Autodesk Fusion 360 part; units mm, degrees
sketch "Esquisse1" plane through (0, 0, 0) normal (0, 0, 1) x (1, 0, 0)
  line L0 (-37.7016, 28.5178) -> (39.7984, 28.5178)
  line L1 (39.7984, 28.5178) -> (39.7984, -27.4822)
  line L2 (39.7984, -27.4822) -> (-37.7016, -27.4822)
  line L3 (-37.7016, -27.4822) -> (-37.7016, 28.5178)
  dimension "d1" = 77.5
  dimension "d2" = 56
extrude "Extrusion1" add sketch "Esquisse1" along normal blind 19
sketch "Esquisse2" plane through (0, 0, 19) normal (0, 0, 1) x (-1, 0, 0)
  line L0 (37.7016, 27.4822) -> (-39.7984, 27.4822)
  line L1 (-39.7984, 27.4822) -> (-39.7984, -28.5178)
  line L2 (-39.7984, -28.5178) -> (37.7016, -28.5178)
  line L3 (37.7016, -28.5178) -> (37.7016, 27.4822)
  line L4 (-39.2984, -28.0178) -> (37.2016, -28.0178)
  line L5 (37.2016, -28.0178) -> (37.2016, 26.9822)
  line L6 (37.2016, 26.9822) -> (-39.2984, 26.9822)
  line L7 (-39.2984, 26.9822) -> (-39.2984, -28.0178)
  dimension "d5" = -0.5
extrude "Extrusion2" cut sketch "Esquisse2" against normal blind 15 contours L4 L5 L6 L7
sketch "Esquisse5" plane through (0, 0, 4) normal (0, 0, 1) x (-1, 0, 0)
  line L0 (-39.2984, 26.9822) -> (-39.2984, -28.0178)
  line L1 (-39.2984, -28.0178) -> (37.2016, -28.0178)
  line L2 (37.2016, -28.0178) -> (37.2016, 26.9822)
  line L3 (37.2016, 26.9822) -> (-39.2984, 26.9822)
  line L4 (37.7016, 27.4822) -> (-39.7984, 27.4822)
  line L5 (-39.2984, 26.9822) -> (37.2016, 26.9822)
  line L6 (37.2016, -28.0178) -> (-39.2984, -28.0178)
  line L7 (-39.7984, -28.5178) -> (37.7016, -28.5178)
  line L8 (-24.7984, 27.4822) -> (-11.7984, 27.4822)
  line L9 (-11.7984, 27.4822) -> (-11.7984, 26.9822)
  line L10 (-11.7984, 26.9822) -> (-24.7984, 26.9822)
  line L11 (-24.7984, 26.9822) -> (-24.7984, 27.4822)
  line L12 (9.7016, -28.0178) -> (22.7016, -28.0178)
  line L13 (22.7016, -28.0178) -> (22.7016, -28.5178)
  line L14 (22.7016, -28.5178) -> (9.7016, -28.5178)
  line L15 (9.7016, -28.5178) -> (9.7016, -28.0178)
  line L16 (-39.7984, 27.4822) -> (-39.7984, -28.5178)
  line L17 (-39.2984, -28.0178) -> (-39.2984, 26.9822)
  line L18 (37.2016, 26.9822) -> (37.2016, -28.0178)
  line L19 (37.7016, -28.5178) -> (37.7016, 27.4822)
  dimension "d11" = 13
  dimension "d12" = 13
  dimension "d13" = 15
  dimension "d14" = 15
extrude "Extrusion3" add sketch "Esquisse5" along normal blind 16.5 contours L3 L4 L5 L8 L9 L10 L11 | L1 L6 L7 L12 L13 L14 L15
sketch "Esquisse6" plane through (0, 0, 4) normal (0, 0, 1) x (-1, 0, 0)
  line L0 (-39.2984, 26.9822) -> (-39.2984, -28.0178)
  line L1 (-39.2984, -28.0178) -> (37.2016, -28.0178)
  line L2 (37.2016, -28.0178) -> (37.2016, 26.9822)
  line L3 (37.2016, 26.9822) -> (-39.2984, 26.9822)
  circle A0 centre (14.7016, -24.5178) radius 1
  circle A1 centre (17.2016, 23.4822) radius 1
  line L4 (37.7016, -28.5178) -> (37.7016, 27.4822)
  line L5 (9.7016, -28.5178) -> (22.7016, -28.5178)
  line L6 (37.7016, 27.4822) -> (-11.7984, 27.4822)
  dimension "d17" = 2
  dimension "d18" = 2
  dimension "d22" = 4
  dimension "d23" = 4
  dimension "d49" = 20
  dimension "d50" = 22.5
extrude "Extrusion4" add sketch "Esquisse6" along normal blind 6 contours A0 | A1
sketch "Esquisse7" plane through (-37.7016, 0, 0) normal (-1, 0, 0) x (0, -1, 0)
  line L0 (-28.5178, 0) -> (27.4822, 0)
  line L1 (27.4822, 0) -> (27.4822, 19)
  line L2 (27.4822, 19) -> (-28.5178, 19)
  line L3 (-28.5178, 19) -> (-28.5178, 0)
  line L4 (-18.5178, 10.6) -> (-6.5178, 10.6)
  line L5 (-6.5178, 10.6) -> (-6.5178, 3.1)
  line L6 (-6.5178, 3.1) -> (-18.5178, 3.1)
  line L7 (-18.5178, 3.1) -> (-18.5178, 10.6)
  line L8 (13.4822, 17.1) -> (21.9822, 17.1)
  line L9 (21.9822, 17.1) -> (21.9822, 4.1)
  line L10 (21.9822, 4.1) -> (13.4822, 4.1)
  line L11 (13.4822, 4.1) -> (13.4822, 17.1)
  dimension "d26" = 12
  dimension "d27" = 7.5
  dimension "d28" = 10
  dimension "d29" = 8.5
  dimension "d30" = 13
  dimension "d31" = 5.5
  dimension "d32" = 4.1
  dimension "d33" = 3.1
extrude "Extrusion5" cut sketch "Esquisse7" against normal blind 33 contours L4 L5 L6 L7 | L8 L9 L10 L11
extrude "Extrusion6" cut sketch "Esquisse6" against normal blind 3
extrude "Extrusion7" add 1 faces at (-11.8683, 9.8511, 0) along direction (0, 0, -1) blind 2
sketch "Esquisse8" plane through (0, 0, 0) normal (0, 0, 1) x (1, 0, 0)
  line L0 (39.7984, 28.5178) -> (-9.7016, 28.5178)
  line L1 (-9.7016, 28.5178) -> (-22.7016, 28.5178)
  line L2 (-22.7016, 28.5178) -> (-37.7016, 28.5178)
  line L3 (-37.7016, 28.5178) -> (-37.7016, -27.4822)
  line L4 (39.7984, -27.4822) -> (39.7984, 28.5178)
  line L5 (24.7984, -27.4822) -> (39.7984, -27.4822)
  line L6 (11.7984, -27.4822) -> (24.7984, -27.4822)
  line L7 (-37.7016, -27.4822) -> (11.7984, -27.4822)
  line L8 (24.7984, -29.4822) -> (41.7984, -29.4822)
  line L9 (41.7984, -29.4822) -> (41.7984, 30.5178)
  line L10 (41.7984, 30.5178) -> (-9.7016, 30.5178)
  line L11 (-9.7016, 30.5178) -> (-22.7016, 30.5178)
  line L12 (-22.7016, 30.5178) -> (-39.7016, 30.5178)
  line L13 (-39.7016, 30.5178) -> (-39.7016, -29.4822)
  line L14 (-39.7016, -29.4822) -> (11.7984, -29.4822)
  line L15 (11.7984, -29.4822) -> (24.7984, -29.4822)
  dimension "d40" = 2
extrude "Extrusion8" add sketch "Esquisse8" along normal blind 24 and the other way blind 2
extrude "Extrusion9" cut 2 faces at (-37.7016, -16.3155, 8.4333) (-37.7016, 14.5178, 5.6) along direction (1, 0, 0) blind 0 and the other way blind 5
extrude "Extrusion10" add sketch "Esquisse6" along normal blind 6 and the other way blind 2 contours A1
sketch "Esquisse9" plane through (39.7984, 0, 0) normal (-1, 0, 0) x (0, -1, 0)
  line L0 (-28.5178, 19) -> (27.4822, 19)
  line L1 (27.4822, 19) -> (27.4822, 24)
  line L2 (27.4822, 24) -> (-28.5178, 24)
  line L3 (-28.5178, 24) -> (-28.5178, 19)
  line L4 (12.4822, 24) -> (22.4822, 24)
  line L5 (22.4822, 24) -> (22.4822, 23.3)
  line L6 (22.4822, 23.3) -> (12.4822, 23.3)
  line L7 (12.4822, 23.3) -> (12.4822, 24)
  dimension "d55" = 10
  dimension "d56" = 0.7
  dimension "d57" = 5
extrude "Extrusion11" add sketch "Esquisse9" along normal blind 2 contours L2 L4 L5 L6 L7
sketch "Esquisse10" plane through (-37.7016, 0, 0) normal (1, 0, 0) x (0, 1, 0)
  line L0 (-27.4822, 19) -> (28.5178, 19)
  line L1 (28.5178, 19) -> (28.5178, 24)
  line L2 (28.5178, 24) -> (-27.4822, 24)
  line L3 (-27.4822, 24) -> (-27.4822, 19)
  line L4 (-27.4822, 24) -> (-17.4822, 24)
  line L5 (-17.4822, 24) -> (-17.4822, 23.3)
  line L6 (-17.4822, 23.3) -> (-27.4822, 23.3)
  line L7 (-27.4822, 23.3) -> (-27.4822, 24)
  dimension "d60" = 10
  dimension "d61" = 0.7
extrude "Extrusion12" add sketch "Esquisse10" along normal blind 2 contours L2 L3 L4 L5 L6 L7
fillet "Congé1" radius 0.45 4 edges at (41.7984, -29.4822, 11) (41.7984, 30.5178, 11) (-39.7016, 30.5178, 11) (-39.7016, -29.4822, 11)
equation "d1 = LongueurBoite"
equation "d2 = LargeurBoite"
equation "d26 = LargeurTrouUSB"
equation "d27 = HauteurTrouUSB"
equation "d28 = DistanceBordTrouUSB"
equation "d29 = LargeurTrouAC"
equation "d30 = HauteurTrouAC"
equation "d31 = DistanceBordTrouAC"
equation "d32 = DistanceDessousTrouAC"
equation "d33 = DistanceDessousTrouUSB"
equation "LargeurBoite = 56 mm"
equation "LongueurBoite = 77.5 mm"
equation "LargeurTrouAC = 8.5 mm"
equation "HauteurTrouAC = 13 mm"
equation "LargeurTrouUSB = 12 mm"
equation "HauteurTrouUSB = 7.5 mm"
equation "DistanceBordTrouUSB = 10 mm"
equation "DistanceBordTrouAC = 5.5 mm"
equation "DistanceDessousTrouUSB = 3.1 mm"
equation "DistanceDessousTrouAC = 4.1 mm"
Here's how the part is built. I have some questions about the finished solid (model axes, mm). A direction names the side the tool comes from. Round coordinates to 2 decimals unless told otherwise and drop trailing zeros. Write each loop counter-clockwise with the first axis right and the second up, starting at its lowest first coordinate (ties: lowest second). Pieces come first, ordered by that corner, then holes.
Q1. If we mould it in two halves opening along X, with no side actions, what happens to faces 5 (the flat face through (-39.702, 1, 11)), 6 (the flat face through (39.798, 0, 21)), 7 (the flat face through (-38, -18, 17.1))? For each: +X half, -X half, draft (parallel to the pull), parting line (faces both ways), or undercut.
Q2. If we section it at C-C on z = 6.5: Write out the boundary of the cut face in (x, y).
Q3. Will these pins go through, and if not, where does the flat tip stop? P1, Ø1.6, axis at x = -17, y = -24, coming from the +Z side; P2, Ø16.5, axis at x = -6.5, y = 13, coming from the +Z side.
Q4. If we section it at B-B on x = 13.5: Write out the boundary of the cut face in (y, z), plus the area to 3 significant figures.
Q5. Which directions (+Z, -Z, +X, -X, +Y, -Y) give clear straight access to the entire face, cutting with the end or side of a thin tool? Please do faces 1 (the flat face through (-38, 18.518, 7)), 2 (the cylindrical face through (-13.965, 23.842, 5.563)), 3 (the flat face through (2, 30.518, 11)), 4 (the flat face through (-37, -22, 23.3)).
Q6. If we section it at D-D on z = 18: Write out the boundary of the cut face in (x, y), plus the area to 3 significant figures.
Q7. If we section it at A-A on y = 8: Write out the boundary of the cut face in (x, z).
Q8. Please list where these lines run through material, in increasing order: probe 1 along Y at (x, z) = (24, 21); probe 2 along X at (y, z) = (-8, 5.5); probe 3 along Y at (x, z) = (-14.5, 6.75).
Answer below:
1. face 5: -X half
1. face 6: undercut
1. face 7: draft
2. outline: (-39.7, -29.03) arc R0.45 ccw to (-39.25, -29.48) - (41.35, -29.48) arc R0.45 ccw to (41.8, -29.03) - (41.8, 30.07) arc R0.45 ccw to (41.35, 30.52) - (-39.25, 30.52) arc R0.45 ccw to (-39.7, 30.07) - (-39.7, 18.52) - (-37.2, 18.52) - (-37.2, 28.02) - (39.3, 28.02) - (39.3, -26.98) - (-37.2, -26.98) - (-37.2, -21.98) - (-39.7, -21.98) - close; (-39.7, -13.48) - (-37.2, -13.48) - (-37.2, 6.52) - (-39.7, 6.52) - close; circle Ø2 at (-17.2, -23.48); circle Ø2 at (-14.7, 24.52)
3. P1: stops at z = 10
3. P2: stops at z = 1
4. outline: (-29.48, -2) - (30.52, -2) - (30.52, 24) - (28.52, 24) - (28.52, 19) - (28.02, 19) - (28.02, 1) - (-26.98, 1) - (-26.98, 20.5) - (-27.48, 20.5) - (-27.48, 24) - (-29.48, 24) - close
4. area: 291 mm2
5. face 1: -X
5. face 2: +Z
5. face 3: +Z, -Z, +X, -X, +Y
5. face 4: none
6. outline: (-39.7, -29.03) arc R0.45 ccw to (-39.25, -29.48) - (41.35, -29.48) arc R0.45 ccw to (41.8, -29.03) - (41.8, 30.07) arc R0.45 ccw to (41.35, 30.52) - (-39.25, 30.52) arc R0.45 ccw to (-39.7, 30.07) - close; hole (-37.2, -26.98) - (39.3, -26.98) - (39.3, 28.02) - (-37.2, 28.02) - close
6. area: 682 mm2
7. outline: (-39.7, -2) - (41.8, -2) - (41.8, 24) - (39.8, 24) - (39.8, 19) - (39.3, 19) - (39.3, 1) - (-37.2, 1) - (-37.2, 3.1) - (-39.7, 3.1) - close; (-39.7, 10.6) - (-37.2, 10.6) - (-37.2, 19) - (-37.7, 19) - (-37.7, 24) - (-39.7, 24) - close
8. probe 1: y = -29.48 to -27.48, 28.52 to 30.52
8. probe 2: x = -39.7 to -37.2, 39.3 to 41.8
8. probe 3: y = -29.48 to -26.98, 23.54 to 25.5, 28.02 to 30.52
